Here's how the part is built. I have some questions about the finished solid (model axes, mm). A direction names the side the tool comes from. Round coordinates to 2 decimals unless told otherwise and drop trailing zeros. Order: outer loops, then holes, each group sorted by start corner. A loop starts at its lowest first (then second) coordinate and runs counter-clockwise, first axis right, second up.
```python
from build123d import *

# Parameters (mm, degrees)
PAD_DEPTH              = 226
POCKET_DEPTH           = 45.978705
POCKET_DEPTH_BACK      = 45.978705
LINEARPATTERN_COUNT    = 4
LINEARPATTERN_PITCH    = 33
LINEARPATTERN001_COUNT = 4
LINEARPATTERN001_PITCH = 33


with BuildPart() as part:
    # Sketch → Pad (new body)
    with BuildSketch(Plane.XY):
        Polygon((45.977705, 111), (-45.977705, 111), (-14.497475, 35), (14.497475, 35), align=None)
    extrude(amount=PAD_DEPTH)

    # Sketch001 → Pocket (cut, two sides)
    with BuildSketch(Plane.YZ) as pocket_sk:
        with BuildLine():
            ThreePointArc((0, 93.52), (-3.52, 90), (0, 86.48))
            Line((0, 86.48), (41.5, 86.48))
            ThreePointArc((41.5, 86.48), (45.02, 90), (41.5, 93.52))
            Line((0, 93.52), (41.5, 93.52))
        make_face()
    pocket = extrude(amount=-POCKET_DEPTH, mode=Mode.SUBTRACT) + extrude(pocket_sk.sketch, amount=POCKET_DEPTH_BACK, mode=Mode.SUBTRACT)

    # LinearPattern: Pocket ×4
    with Locations(*[(0, 0, i * LINEARPATTERN_PITCH) for i in range(1, LINEARPATTERN_COUNT)]):
        add(pocket, mode=Mode.SUBTRACT)

    # Sketch002 → Groove (revolve, cut)
    with BuildSketch(Plane.YZ):
        Polygon((35, 90), (111, 90), (111, 92), (46.02, 92), (46.02, 95), (35, 95), align=None)
    groove = revolve(axis=Axis((0, 35, 90), (0, 1, 0)), mode=Mode.SUBTRACT)

    # LinearPattern001: Groove ×4
    with Locations(*[(0, 0, i * LINEARPATTERN001_PITCH) for i in range(1, LINEARPATTERN001_COUNT)]):
        add(groove, mode=Mode.SUBTRACT)


solid = part.part
```
1. If we section it at B-B, the plane y = 93.5: Write out the boundary of the cut face in (x, z), and give its area (3 significant figures).
Evaluation:
outline: (-38.73, 0) - (38.73, 0) - (38.73, 226) - (-38.73, 226) - close; hole circle Ø4 at (0, 90); hole circle Ø4 at (0, 123); hole circle Ø4 at (0, 156); hole circle Ø4 at (0, 189)
area: 17,500 mm2
2. I'm going to push flat-ended pins straight in: P1, Ø2.5, axis at x = 0, z = 156, coming from the +Y side; P2, Ø3, axis at x = -2, z = 155, coming from the -Y side; P3, Ø5, axis at y = 72, z = 168, coming from the -X side. Where does each tip first touch, or does it pass through?
Evaluation:
P1: passes through
P2: stops at y = 46.02
P3: stops at x = -30.86
3. If we section it at D-D, the plane y = 106: Write out the boundary of the cut face in (x, z), and give its area (3 significant figures).
Evaluation:
outline: (-43.91, 0) - (43.91, 0) - (43.91, 226) - (-43.91, 226) - close; hole circle Ø4 at (0, 90); hole circle Ø4 at (0, 123); hole circle Ø4 at (0, 156); hole circle Ø4 at (0, 189)
area: 19,800 mm2
4. If we mould it in two halves opening along X, with no side actions, what happens to faces 4 (the flat face through (-2.2, 46.02, 90.1)), 5 (the flat face through (10, 38, 126.52))? For each: released by +X, released by -X, zero draft, split by the parting line, or undercut.
Evaluation:
face 4: undercut
face 5: zero draft
5. If we section it at A-A, the plane x = 11: Write out the boundary of the cut face in (y, z), and give its area (3 significant figures).
Evaluation:
outline: (35, 0) - (111, 0) - (111, 226) - (35, 226) - (35, 192.52) - (41.5, 192.52) arc R3.52 cw to (41.5, 185.48) - (35, 185.48) - (35, 159.52) - (41.5, 159.52) arc R3.52 cw to (41.5, 152.48) - (35, 152.48) - (35, 126.52) - (41.5, 126.52) arc R3.52 cw to (41.5, 119.48) - (35, 119.48) - (35, 93.52) - (41.5, 93.52) arc R3.52 cw to (41.5, 86.48) - (35, 86.48) - close
area: 16,900 mm2
6. I need wall thicknesses on probe 1 along Z at (x, y) = (0, 38); probe 2 along X at (y, z) = (41.5, 12.5); probe 3 along Y at (x, z) = (13, 189). Which ranges of each line are inside material? Lowest first, please.
Evaluation:
probe 1: z = 0 to 85, 95 to 118, 128 to 151, 161 to 184, 194 to 226
probe 2: x = -17.19 to 17.19
probe 3: y = 45.02 to 111
7. On a 3-axis mill with a long thin cutter (end or side, diameter ignored), from which of +Z, -Z, +X, -X, +Y, -Y can I reach the whole of each face in a straight line? I mean faces 1 (the flat face through (0, 35, 172)), 2 (the cylindrical face through (0, 40, 151)), 3 (the flat face through (10, 38, 159.52)). Say none if no direction works.
Evaluation:
face 1: +Z, -Z, +X, -X, -Y
face 2: -Y
face 3: +X, -X, -Y
8. If we section it at C-C, the plane z = 98: Write out the boundary of the cut face in (x, y).
Evaluation:
outline: (-45.98, 111) - (-14.5, 35) - (14.5, 35) - (45.98, 111) - close
